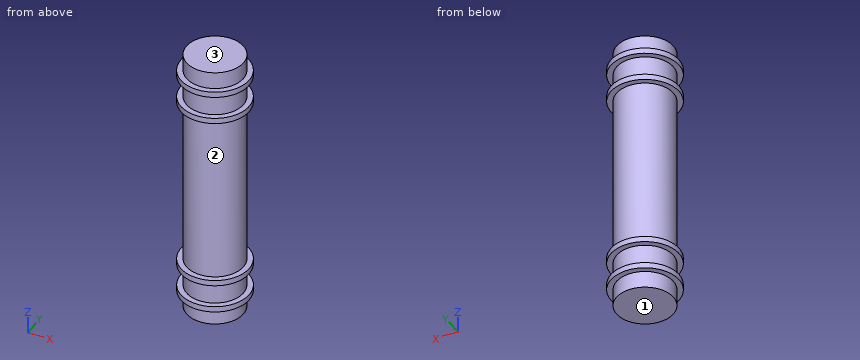
from build123d import *

# Parameters (mm, degrees)
ESBO_O1_R                = 2.5
RESSALTO_EXTRUS_O1_DEPTH = 24
ESBO_O2_W                = 0.5
ESBO_O2_H                = 3
ESBO_O4_W                = 0.5
ESBO_O4_H                = 3


with BuildPart() as part:
    # Esboço1 → Ressalto-extrusão1 (new body)
    with BuildSketch(Plane.XY):
        Circle(ESBO_O1_R)
    extrude(amount=RESSALTO_EXTRUS_O1_DEPTH)

    # Esboço2 → Revolução1 (revolve)
    with BuildSketch(Plane(origin=(0, 0, 0), x_dir=(0, 0, -1), z_dir=(1, 0, 0)), mode=Mode.PRIVATE) as revolu_o1_sk:
        with Locations((-1.75, -1.5)):
            Rectangle(ESBO_O2_W, ESBO_O2_H)
        with Locations((-4.25, -1.5)):
            Rectangle(ESBO_O2_W, ESBO_O2_H)
    revolve(revolu_o1_sk.sketch.rotate(Axis((0, 0, 2), (0, 0, -1)), 270), axis=Axis((0, 0, 2), (0, 0, -1)))

    # Esboço4 → Revolução2 (revolve)
    with BuildSketch(Plane(origin=(0, 0, 0), x_dir=(0, 0, -1), z_dir=(1, 0, 0)), mode=Mode.PRIVATE) as revolu_o2_sk:
        with Locations((-19.75, -1.5)):
            Rectangle(ESBO_O4_W, ESBO_O4_H)
        with Locations((-22.25, -1.5)):
            Rectangle(ESBO_O4_W, ESBO_O4_H)
    revolve(revolu_o2_sk.sketch.rotate(Axis((0, 0, 20), (0, 0, -1)), 90), axis=Axis((0, 0, 20), (0, 0, -1)))


solid = part.part
The listing builds one solid part. Answer for the finished solid, in the listing's coordinates (mm). Face numbers are marked on the shaded views. Coordinates: 2 decimals unless noted, no trailing zeros. Write each loop counter-clockwise with the first axis right and the second up, starting at its lowest first coordinate (ties: lowest second). Pieces come first, ordered by that corner, then holes. Notation, with made-up numbers: M 62.5,-9.75 L 99.5,-9.75 A15 cw 99.5,11.25 Z; hole C 81.25,46.5 d1. An arc over 180 degrees is marked long. Put each result on its own line as item: value. Start each with the question number.
1. A cutting plane is placed at A-A on z = 16.5. Write down the section's boundary in (x, y).
2. For a pull along Z with two mould halves and no side action, classify the marked faces 1, 2 and 3 as pulls with the +Z half, pulls with the -Z half, needs draft (parallel to the pull), parting line crosses it, or undercut.
3. Flat-ended cylindrical pins translate along their axes: P1, Ø2, axis at x = 2, z = 7, coming from the -Y side; P2, Ø1.5, axis at x = -0.5, z = 21, coming from the -Y side. Find the tip coordinate at first contact, or state that the pin passes through.
4. Consider line 1 (Z direction, x = -0.4, y = -2.6); line 2 (X direction, y = -0.15, z = 13.5). Determine where each line is inside the solid, lowest interval first. Write a range as from..to.
Resolved:
1. outline: C 0,0 d5
2. face 1: pulls with the -Z half
2. face 2: undercut
2. face 3: pulls with the +Z half
3. P1: stops at y = -2.29
3. P2: stops at y = -2.5
4. line 1: z = 1.5..2, 4..4.5, 19.5..20, 22..22.5
4. line 2: x = -2.5..2.5
